Part model, mm, in its own coordinate system. A direction names the side the tool comes from. Round coordinates to 2 decimals unless told otherwise and drop trailing zeros. Write each loop counter-clockwise with the first axis right and the second up, starting at its lowest first coordinate (ties: lowest second). Pieces come first, ordered by that corner, then holes. Notation, with made-up numbers: M -35,16 L -3,16 A30 cw -3,50 Z; hole C 68,38.25 d11. An arc over 180 degrees is marked long. Answer as a JSON object with one key per item and string values. Group by question number.
1. Which spindle directions (+Z, -Z, +X, -X, +Y, -Y) get a long thin tool onto all of the face, cutting with end or side? Do faces 4 (the face through (-2, 7.75, 0)), 5 (the face through (56, 0, -0.5)). Say none if no direction does.
2. Band-saw the part on C-C, the plane x = -1.5. Write the cut outline in (y, z).
3. Two-plate mould, pull along Y, no slides. Class faces 1 (the face through (120.25, 0.17, 0.04)), 2 (the face through (2, -7, 2.5)), 3 (the face through (-110.115, 0.751, -0.035)): +Y half, -Y half, draft (parallel to the pull), parting line (faces both ways), or undercut.
4. Band-saw the part on B-B, the plane z = 1.1. Write the cut outline in (x, y).
5. Drop flat-ended pins along their axis: pin 1 (8 mm diameter, centred on x = 112.5, y = 0, fed in from +Z); pin 2 (0.9 mm diameter, centred on y = -2, z = 1.5, fed in from +X); pin 3 (6.5 mm diameter, centred on x = -58, y = 2, fed in from +Z); pin 4 (0.9 mm diameter, centred on y = -3, z = 1, fed in from +X). Give the stop position or say it passes through.
6. Drill centre lines: line 1 (Y direction, x = -112.5, z = -0.4); line 2 (Y direction, x = 59, z = 0.15); line 3 (X direction, y = -4.25, z = 2.1). Where is each one in solid material? Low to high. Write a range as from..to.
7. Band-saw the part on A-A, the plane y = 0. Write the cut outline in (x, z), plus the area to 3 significant figures.
from build123d import *

# Parameters (mm, degrees)
CROQUIS1_R              = 2.5
SALIENTE_EXTRUIR1_DEPTH = 2.5
CROQUIS4_W              = 18.2
CROQUIS4_H              = 13.1
CORTAR_EXTRUIR4_DEPTH   = 3


with BuildPart() as part:
    # Croquis1 → Saliente-Extruir1 (new, symmetric)
    with BuildSketch(Plane.XY):
        with BuildLine():
            Line((-112.5, 7.75), (112.5, 7.75))
            ThreePointArc((112.5, 7.75), (120.25, 0), (112.5, -7.75))
            Line((112.5, -7.75), (-112.5, -7.75))
            ThreePointArc((-112.5, -7.75), (-120.25, 0), (-112.5, 7.75))
        make_face()
        with Locations((112.5, 0)):
            Circle(CROQUIS1_R, mode=Mode.SUBTRACT)
        with Locations((-112.5, 0)):
            Circle(CROQUIS1_R, mode=Mode.SUBTRACT)
    extrude(amount=SALIENTE_EXTRUIR1_DEPTH, both=True)

    # Croquis4 → Cortar-Extruir4 (cut)
    with BuildSketch(Plane.XY.offset(2.5)):
        Rectangle(CROQUIS4_W, CROQUIS4_H)
        with Locations((-56.25, 0)):
            Rectangle(CROQUIS4_W, CROQUIS4_H)
        with Locations((56.25, 0)):
            Rectangle(CROQUIS4_W, CROQUIS4_H)
    extrude(amount=-CORTAR_EXTRUIR4_DEPTH, mode=Mode.SUBTRACT)


solid = part.part
Worked answers:
{
 "1": {"face 4": "+Z, -Z, +X, -X, +Y", "face 5": "+Z"},
 "2": {"outline": "M -7.75,-2.5 L 7.75,-2.5 L 7.75,2.5 L 6.55,2.5 L 6.55,-0.5 L -6.55,-0.5 L -6.55,2.5 L -7.75,2.5 Z"},
 "3": {"face 1": "parting line", "face 2": "draft", "face 3": "undercut"},
 "4": {"outline": "M -112.5,-7.75 L 112.5,-7.75 A7.75 ccw 112.5,7.75 L -112.5,7.75 A7.75 ccw Z; hole C -112.5,0 d5; hole M -65.35,-6.55 L -47.15,-6.55 L -47.15,6.55 L -65.35,6.55 Z; hole M -9.1,-6.55 L 9.1,-6.55 L 9.1,6.55 L -9.1,6.55 Z; hole M 47.15,-6.55 L 65.35,-6.55 L 65.35,6.55 L 47.15,6.55 Z; hole C 112.5,0 d5"},
 "5": {"pin 1": "stops at z = 2.5", "pin 2": "stops at x = 120.09", "pin 3": "stops at z = -0.5", "pin 4": "stops at x = 119.82"},
 "6": {"line 1": "y = -7.75..-2.5, 2.5..7.75", "line 2": "y = -7.75..-6.55, 6.55..7.75", "line 3": "x = -118.98..-65.35, -47.15..-9.1, 9.1..47.15, 65.35..118.98"},
 "7": {"outline": "M -120.25,-2.5 L -115,-2.5 L -115,2.5 L -120.25,2.5 Z; M -110,-2.5 L 110,-2.5 L 110,2.5 L 65.35,2.5 L 65.35,-0.5 L 47.15,-0.5 L 47.15,2.5 L 9.1,2.5 L 9.1,-0.5 L -9.1,-0.5 L -9.1,2.5 L -47.15,2.5 L -47.15,-0.5 L -65.35,-0.5 L -65.35,2.5 L -110,2.5 Z; M 115,-2.5 L 120.25,-2.5 L 120.25,2.5 L 115,2.5 Z", "area": "989 mm^2"}
}
